Geometry: final body of the model. Coordinates: model frame, mm. A direction names the side the tool comes from. Coordinates: 2 decimals unless noted, no trailing zeros. Order: outer loops, then holes, each group sorted by start corner. A loop starts at its lowest first (then second) coordinate and runs counter-clockwise, first axis right, second up. Notation, with made-up numbers: M 64.25,71 L 74.25,71 A15 ccw 74.25,77 Z; hole C 72,-21.75 d6. An arc over 180 degrees is marked long. Use CSV: the item, a comma, the result in double quotes. Start each with the question number.
1. Section query B-B on y = -13. Return the cut outline in (x, z), and give its area (3 significant figures).
2. Set-up query: faces 4 (the flat face through (0, 0, 58)), 5 (the cylindrical face through (-4.268, 8.206, 17.748)), 6 (the cylindrical face through (-4.268, 8.206, 37.986)), 7 (the flat face through (8.3, 1.3, 56)). Return all of +Z, -Z, +X, -X, +Y, -Y with unobstructed straight access to the full face (end or side cutting, diameter ignored); none if empty.
3. Material intervals for line 1 (Z direction, x = -13.5, y = 6); line 2 (Y direction, x = -5.5, z = 14.5); line 3 (X direction, y = 8, z = 40.5), sorted ascending.
4. First-contact query: P1, Ø8, axis at x = -3.5, z = 17.5, coming from the -Y side; P2, Ø4, axis at x = -7.5, y = 11.5, coming from the -Z side; P3, Ø3, axis at y = 5.5, z = 37.5, coming from the +X side. Flat tips, straight axial feed; report the tip coordinate or a pass-through.
5. Pull-direction query (Z, two-part tool) for faces 1 (the cylindrical face through (7.62, -3.16, 56.99)), 2 (the flat face through (6.5, 6.9, 36)), 3 (the flat face through (6.5, 6.9, 39)); classes: pulls with the +Z half, pulls with the -Z half, needs draft (parallel to the pull), parting line crosses it, or undercut.
6. Section query D-D on z = 22. Return the cut outline in (x, y), and give its area (3 significant figures).
7. Section query A-A on x = 0. Return the cut outline in (y, z).
8. Section query C-C on x = 11.75. Return the cut outline in (y, z).
from build123d import *

# Parameters (mm, degrees)
SKETCH1_R           = 9.25
BOSS_EXTRUDE1_DEPTH = 58
CUT_EXTRUDE1_START  = -2
SKETCH2_R           = 9.25
SKETCH2_R_2         = 8.25
CUT_EXTRUDE1_DEPTH  = 2
SKETCH3_R           = 15
BOSS_EXTRUDE2_DEPTH = 1
LPATTERN1_COUNT     = 2
LPATTERN1_PITCH     = 3


with BuildPart() as part:
    # Sketch1 → Boss-Extrude1 (new body)
    with BuildSketch(Plane.XY):
        with Locations(Location((0, 0, 0), (0, 0, 180))):
            Circle(SKETCH1_R)
    extrude(amount=BOSS_EXTRUDE1_DEPTH)

    # Sketch2 → Cut-Extrude1 (cut)
    with BuildSketch(Plane.XY.offset(58).offset(CUT_EXTRUDE1_START)):
        with Locations(Location((0, 0, 0), (0, 0, 180))):
            Circle(SKETCH2_R)
        Circle(SKETCH2_R_2, mode=Mode.SUBTRACT)
    extrude(amount=CUT_EXTRUDE1_DEPTH, mode=Mode.SUBTRACT)

    # Sketch3 → Boss-Extrude2 (add)
    with BuildSketch(Plane.XY.offset(36)):
        Circle(SKETCH3_R)
    boss_extrude2 = extrude(amount=BOSS_EXTRUDE2_DEPTH)

    # LPattern1: Boss-Extrude2 ×2
    with Locations(*[(0, 0, i * LPATTERN1_PITCH) for i in range(1, LPATTERN1_COUNT)]):
        add(boss_extrude2)


solid = part.part
Results list:
1,outline,"M -7.48,36 L 7.48,36 L 7.48,37 L -7.48,37 Z; M -7.48,39 L 7.48,39 L 7.48,40 L -7.48,40 Z"
1,area,"29.9 mm²"
2,face 4,"+Z, +X, -X, +Y, -Y"
2,face 5,"-Z"
2,face 6,"none"
2,face 7,"+Z"
3,line 1,"z = 36 to 37, 39 to 40"
3,line 2,"y = -7.44 to 7.44"
3,line 3,"x = -4.64 to 4.64"
4,P1,"stops at y = -9.25"
4,P2,"stops at z = 36"
4,P3,"stops at x = 14.43"
5,face 1,"needs draft"
5,face 2,"pulls with the -Z half"
5,face 3,"undercut"
6,outline,"C 0,0 d18.5"
6,area,"269 mm²"
7,outline,"M -15,36 L -9.25,36 L -9.25,0 L 9.25,0 L 9.25,36 L 15,36 L 15,37 L 9.25,37 L 9.25,39 L 15,39 L 15,40 L 9.25,40 L 9.25,56 L 8.25,56 L 8.25,58 L -8.25,58 L -8.25,56 L -9.25,56 L -9.25,40 L -15,40 L -15,39 L -9.25,39 L -9.25,37 L -15,37 Z"
8,outline,"M -9.32,36 L 9.32,36 L 9.32,37 L -9.32,37 Z; M -9.32,39 L 9.32,39 L 9.32,40 L -9.32,40 Z"
